Autodesk Inventor part; units mm, degrees
ref_plane "Work Plane1" through (0, 0, 71.12) normal (0, 0, 1) x (1, 0, 0)
ref_plane "Work Plane5" through (0, 0, 85.09) normal (0, 0, 1) x (1, 0, 0)
ref_plane "Work Plane8" through (4.445, 0, 85.09) normal (1, 0, 0) x (0, 1, 0)
sketch "Sketch1" plane through (0, 0, 0) normal (0, 0, 1) x (1, 0, 0)
  circle A0 centre (0, 0) radius 7.874
  dimension "d0" = 15.748
extrude "Extrusion1" add sketch "Sketch1" along normal blind 67.31
ref_plane "Work Plane1" through (0, 0, 71.12) normal (0, 0, 1) x (1, 0, 0)
sketch "Sketch3" plane through (0, 0, 71.12) normal (0, 0, 1) x (1, 0, 0)
  circle A0 centre (0, 0) radius 3.81
  dimension "d4" = 7.62
loft "Loft1" add profiles "Sketch3" section 1 edges at (-7.874, 0, 67.31)
ref_plane "Work Plane5" through (0, 0, 85.09) normal (0, 0, 1) x (1, 0, 0)
ref_plane "Work Plane8" through (4.445, 0, 85.09) normal (1, 0, 0) x (0, 1, 0)
sketch "Sketch6" plane through (4.445, 0, 85.09) normal (1, 0, 0) x (0, 1, 0)
  line L0 (4.445, 0) -> (-4.445, 0)
  point P0 (0, -85.09)
  point P1 (0, -4.826)
  dimension "d23" = 4.826
ref_plane "Work Plane6" through (4.445, 0, 85.09) normal (1, 0, 0) x (0, 1, 0)
sketch "Sketch8" plane through (4.445, 0, 85.09) normal (1, 0, 0) x (0, 1, 0)
  line L0 (-5.08, -94.742) -> (5.08, -94.742)
  point P0 (0, -85.09)
  point P1 (0, -89.662)
  dimension "d31" = 5.08
sketch "Sketch9" plane through (0, 0, 0) normal (0, 0, -1) x (-1, 0, 0)
  line L0 (-3.81, 3.81) -> (3.81, 3.81)
  line L1 (3.81, 3.81) -> (3.81, -3.81)
  line L2 (3.81, -3.81) -> (-3.81, -3.81)
  line L3 (-3.81, -3.81) -> (-3.81, 3.81)
  line L4 (-3.81, 3.81) -> (3.81, -3.81) construction
  line L5 (3.81, 3.81) -> (-3.81, -3.81) construction
  point P0 (0, 0)
  dimension "d39" = 7.62
  dimension "d40" = 7.62
extrude "Extrusion6" add sketch "Sketch9" along normal blind 9.652
hole "Hole3" at (4.445, 0, -4.572) direction (-1, 0, 0) diameter 5.08 end through all both
sketch "Sketch10" plane through (0, 0, 71.12) normal (0, 0, 1) x (1, 0, 0)
  line L0 (3.175, 3.81) -> (-3.175, 3.81)
  line L1 (-3.175, 3.81) -> (-3.175, -3.81)
  line L2 (-3.175, -3.81) -> (3.175, -3.81)
  line L3 (3.175, -3.81) -> (3.175, 3.81)
  line L4 (3.175, 3.81) -> (-3.175, -3.81) construction
  line L5 (-3.175, 3.81) -> (3.175, -3.81) construction
  point P0 (0, 0)
  point P1 (0, 0)
  dimension "d50" = 6.35
  dimension "d51" = 7.62
extrude "Extrusion7" add sketch "Sketch10" along normal blind 13.97
hole "Hole4" at (4.445, 0, 80.264) direction (-1, 0, 0) diameter 5.08 end through all
fillet "Fillet1" radius 3.175 2 edges at (0, 3.81, 85.09) (0, -3.81, 85.09)
fillet "Fillet2" radius 3.175 2 edges at (0, 3.81, -9.652) (0, -3.81, -9.652)
properties part number "MockShock2"
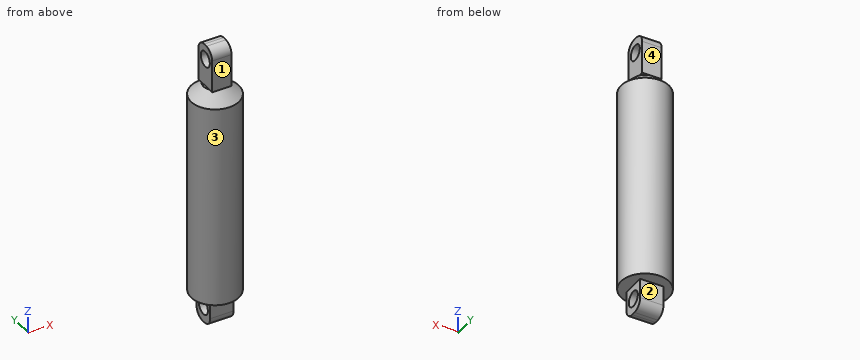
Could you check a few things on this model? Use its own coordinates, in mm. Face numbers are marked on the shaded views. A direction names the side the tool comes from. Give positions to 0.01 mm unless a question says otherwise; leave off trailing zeros. Order: outer loops, then holes, each group sorted by start corner. A loop starts at its lowest first (then second) coordinate and runs counter-clockwise, first axis right, second up. Notation, with made-up numbers: (-16, -3.5) -> (23, -3.5) arc R5 cw to (23, 5.5) -> close; hole circle Ø4 at (-26.5, 15.25). An arc over 180 degrees is marked (long way). Answer in a Markdown table with one row per item. Add a question column.
Item 1: Imagine slicing it at A-A (z = 26.5). List the corners of the cut face in (x, y) for me, and give its area (3 significant figures).
Item 2: Please list where these lines run through material, in increasing order: probe 1 along Z at (x, y) = (1.5, 0); probe 2 along Z at (x, y) = (2.75, 1.75); probe 3 along Z at (x, y) = (-3.25, 1).
Item 3: For the marked faces 1, 2, 3 and 4, which set-ups out of +Z, -Z, +X, -X, +Y, -Y let a thin tool reach every point of the face, with its end or its side?
Item 4: I'm going to push flat-ended pins straight in: P1, Ø4, axis at x = 6, y = -2, coming from the +Z side; P2, Ø1.9, axis at x = 0, z = -3, coming from the -Y side; P3, Ø0.9, axis at x = 1.5, y = -3, coming from the -Z side. Where does each tip first touch, or does it pass through?
Result:
| question | item | result |
|---|---|---|
| 1 | outline | circle Ø15.75 at (0, 0) |
| 1 | area | 195 mm2 |
| 2 | probe 1 | -9.65 to -7.11, -2.03 to 77.72, 82.8 to 85.09 |
| 2 | probe 2 | -9.45 to -6.41, -2.73 to 78.42, 82.1 to 84.89 |
| 2 | probe 3 | -9.63 to -6.91, -2.24 to 71.12 |
| 3 | face 1 | +Z, +X, -X, -Y |
| 3 | face 2 | -Z, +X, -X, +Y |
| 3 | face 3 | +Z, -Z |
| 3 | face 4 | +Z, +X, -X, +Y |
| 4 | P1 | z = 70.64 |
| 4 | P2 | y = -3.81 |
| 4 | P3 | z = -9.01 |
